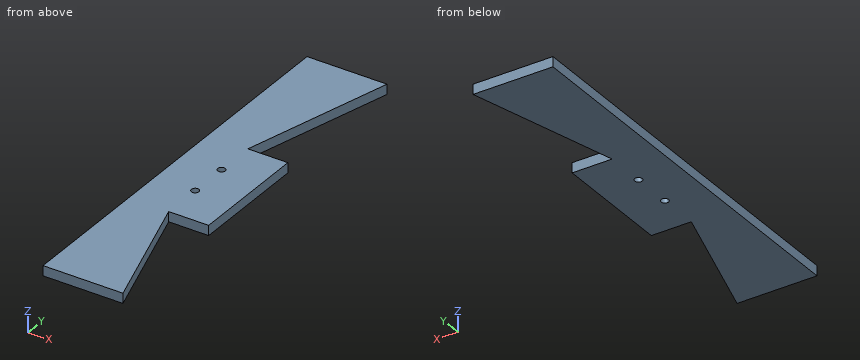
from build123d import *

# Parameters (mm, degrees)
F1_DEPTH = 19.05
F0_R     = 9.525
F2_DEPTH = 25.4


with BuildPart() as f1:
    # F0 (on Top) → F1 (new body)
    with BuildSketch(Plane.XY):
        Polygon((154.2242345231, 0), (52.7512345231, 0), (52.7512345231, -381.426606369), (154.3512345231, -381.426606369), (255.9512345231, 0), align=None)
    extrude(amount=F1_DEPTH)

    # F0 (on Top) → F2 (join)
    with BuildSketch(Plane.XY):
        Polygon((154.2242345231, 0), (52.7512345231, 0), (52.7512345231, -381.426606369), (154.3512345231, -381.426606369), (255.9512345231, 0), align=None)
        Polygon((154.3512345231, -686.226606369), (52.7512345231, -686.226606369), (52.7512345231, -1016), (154.2242345231, -1016), (255.9512345231, -1016), align=None)
        Polygon((154.3512345231, -381.426606369), (52.7512345231, -381.426606369), (52.7512345231, -686.226606369), (154.3512345231, -686.226606369), (255.9512345231, -686.226606369), (255.9512345231, -381.426606369), align=None)
        with Locations((154.2242345231, -584.2)):
            Circle(F0_R, mode=Mode.SUBTRACT)
        with Locations((154.2242345231, -482.6)):
            Circle(F0_R, mode=Mode.SUBTRACT)
    extrude(amount=F2_DEPTH)


solid = f1.part
Could you check a few things on this model? Use its own coordinates, in mm. Coordinates: 2 decimals unless noted, no trailing zeros. Write each loop counter-clockwise with the first axis right and the second up, starting at its lowest first coordinate (ties: lowest second). Pieces come first, ordered by that corner, then holes. Notation, with made-up numbers: (62.5, 67.25) - (96.5, 67.25) arc R19 cw to (96.5, 73.25) - close; hole circle Ø11 at (6.25, -13.5). An arc over 180 degrees is marked (long way). Put each result on its own line as item: value. Start each with the question number.
Q1. I want a section at D-D on y = -113. Write out the boundary of the cut face in (x, z), plus the area to 3 significant figures.
Q2. I want a section at A-A on y = -584.2. Write out the boundary of the cut face in (x, z).
Q3. I want a section at B-B on z = 21.5. Write out the boundary of the cut face in (x, y) (3 decimals).
Q4. I want a section at C-C on x = 183. Write out the boundary of the cut face in (y, z).
Q5. I'm going to push a flat-ended pin straight in: P1, Ø3, axis at y = -192.5, z = 21.5, coming from the +X side. Where does the tip first touch, or does it pass through?
Q6. Please list where these lines run through material, in increasing order: L1, parallel to X at y = -584.2, z = 15.75; L2, parallel to X at y = -177, z = 9; L3, parallel to X at y = -825, z = 21.75.
Checks:
1. outline: (52.75, 0) - (225.85, 0) - (225.85, 25.4) - (52.75, 25.4) - close
1. area: 4,400 mm²
2. outline: (52.75, 0) - (144.7, 0) - (144.7, 25.4) - (52.75, 25.4) - close; (163.75, 0) - (255.95, 0) - (255.95, 25.4) - (163.75, 25.4) - close
3. outline: (52.751, -1016) - (255.951, -1016) - (154.351, -686.227) - (255.951, -686.227) - (255.951, -381.427) - (154.351, -381.427) - (255.951, 0) - (52.751, 0) - close; hole circle Ø19.05 at (154.224, -584.2); hole circle Ø19.05 at (154.224, -482.6)
4. outline: (-1016, 0) - (-779.21, 0) - (-779.21, 25.4) - (-1016, 25.4) - close; (-686.23, 0) - (-381.43, 0) - (-381.43, 25.4) - (-686.23, 25.4) - close; (-273.87, 0) - (0, 0) - (0, 25.4) - (-273.87, 25.4) - close
5. P1: x = 205.07
6. L1: 52.75 to 144.7, 163.75 to 255.95
6. L2: 52.75 to 208.8
6. L3: 52.75 to 197.11
